Geometry check sheet. Reference: drawing and pictorial views, mm from the part's lowest x, y, z. A direction names the side the tool comes from. Give positions to 0.01 mm unless a question says otherwise; leave off trailing zeros. Order: outer loops, then holes, each group sorted by start corner. A loop starts at its lowest first (then second) coordinate and runs counter-clockwise, first axis right, second up.
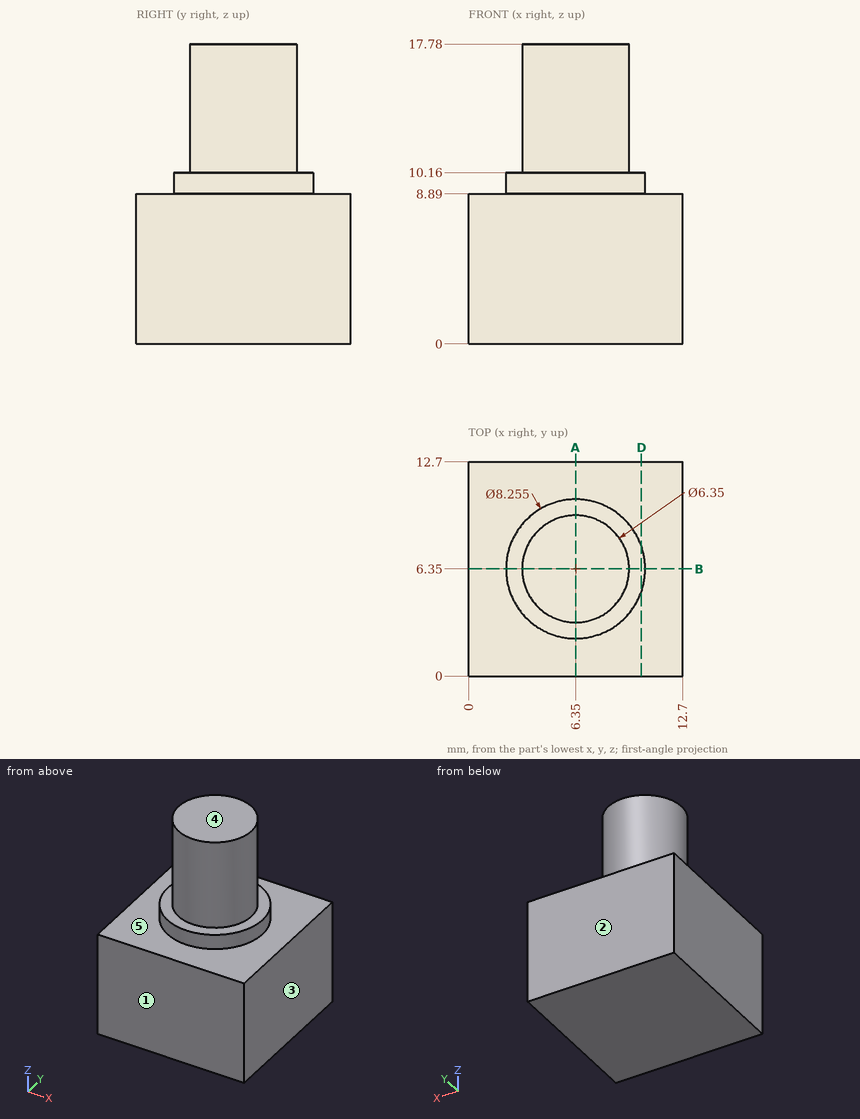
(1) Set-up check for the marked faces 4 and 5: record each of +Z, -Z, +X, -X, +Y, -Y from which the full face is reachable in a straight line by a thin tool's end or side.
Response values:
face 4: +Z, +X, -X, +Y, -Y
face 5: +Z
(2) Gauge pin test, flat ends, axial feed: pin 1 Ø1 at (x, y) = (8.5, 10.5) entering from +Z; pin 2 Ø6 at (y, z) = (4, 11) entering from +X; pin 3 Ø6 at (x, z) = (10, 13.5) entering from -Y; pin 4 Ø6 at (y, z) = (7, 12.5) entering from +X. Record the tip position at first contact, or that the pin passes through.
Response values:
pin 1: stops at z = 8.89
pin 2: stops at x = 12.7
pin 3: stops at y = 3.24
pin 4: stops at x = 10.48
(3) Cross-section at A-A on x = 6.35. Enter the section's corners in (y, z) (1 decimal).
Response values:
outline: (0, 0) - (12.7, 0) - (12.7, 8.9) - (10.5, 8.9) - (10.5, 10.2) - (9.5, 10.2) - (9.5, 17.8) - (3.2, 17.8) - (3.2, 10.2) - (2.2, 10.2) - (2.2, 8.9) - (0, 8.9) - close
(4) Cross-section at D-D on x = 10.25. Enter the section's corners in (y, z).
Response values:
outline: (0, 0) - (12.7, 0) - (12.7, 8.89) - (7.7, 8.89) - (7.7, 10.16) - (5, 10.16) - (5, 8.89) - (0, 8.89) - close
(5) Release check for a two-part mould opening along Y. For the marked faces 1, 2 and 3 record: released by +Y, released by -Y, zero draft, split by the parting line, or undercut.
Response values:
face 1: released by -Y
face 2: released by +Y
face 3: zero draft
(6) Material ranges on L1, parallel to Z at x = 2, y = 8.75; L2, parallel to X at y = 6.5, z = 11.5; L3, parallel to Z at x = 3.5, y = 8.75, recorded low to high.
Response values:
L1: z = 0 to 8.89
L2: x = 3.18 to 9.52
L3: z = 0 to 10.16
